CAD build for the part. Positions are in the model's coordinates, mm. A direction names the side the tool comes from. Coordinates: 2 decimals unless noted, no trailing zeros. Write each loop counter-clockwise with the first axis right and the second up, starting at its lowest first coordinate (ties: lowest second). Pieces come first, ordered by that corner, then holes. Notation, with made-up numbers: (-29.5, 58.25) - (25.5, 58.25) arc R34 ccw to (25.5, 91.25) - close; hole circle Ø10 at (11.5, 10). An arc over 180 degrees is marked (long way). Answer in a Markdown table with one row per item. Add a question column.
Q1. Band-saw the part on A-A (y = 30). List the corners of the cut face in (x, z), and give its area (3 significant figures).
Q2. Pin check, flat tip, straight feed: pin 1 (7.5 mm diameter, centred on x = 22.5, y = 19, fed in from +Z). Stop position of the tip, or through.
Q3. 3-axis set-ups, long thin cutter, end or side, ignore diameter. For faces 4 (the flat face through (0, 17, 2)), 5 (the flat face through (20, 11.5, 1)), 6 (the flat face through (20, 18, 0)), 7 (the cylindrical face through (7, 17, 2)), 8 (the flat face through (31.5, 15.4, 2.5)): which of +Z, -Z, +X, -X, +Y, -Y reach the whole face in a straight line?
Q4. Band-saw the part on C-C (z = 0.45). List the corners of the cut face in (x, y).
Q5. Drill centre lines: line 1 along X through (y, z) = (7, 3.1); line 2 along Y through (x, z) = (22.5, 2.7); line 3 along X through (y, z) = (16, 3.2). Where is each one in solid material? Low to high. Write a range as from..to.
Q6. Two-plate mould, pull along Y, no slides. Class faces 1 (the flat face through (41, 17, 2)), 2 (the cylindrical face through (39.859, 33.797, 2.028)), 3 (the flat face through (20, 19, 2)): +Y half, -Y half, draft (parallel to the pull), parting line (faces both ways), or undercut.
Q7. Band-saw the part on D-D (y = 25). List the corners of the cut face in (x, z), and give its area (3 significant figures).
Q8. Band-saw the part on B-B (x = 13.5). List the corners of the cut face in (y, z), and give its area (3 significant figures).
```python
from build123d import *

# Parameters (mm, degrees)
ESQUISSE1_W             = 41
ESQUISSE1_H             = 35
BOSS_EXTRU_1_DEPTH      = 4
ESQUISSE2_W             = 22
ESQUISSE2_H             = 18
ENL_V_MAT_EXTRU_1_DEPTH = 2
ESQUISSE3_W             = 4
ESQUISSE3_H             = 30
ESQUISSE3_W_2           = 22
ESQUISSE3_H_2           = 3
ENL_V_MAT_EXTRU_2_DEPTH = 6
CONG_4_R                = 4
CONG_6_RADIUS           = 2
CONG_6_LENGTH           = 30
CONG_7_RADIUS           = 2
CONG_7_LENGTH           = 30
CONG_8_RADIUS           = 2
CONG_8_LENGTH           = 30
CONG_9_RADIUS           = 2
CONG_9_LENGTH           = 30


with BuildPart() as part:
    # Esquisse1 → Boss.-Extru.1 (new body)
    with BuildSketch(Plane.XY):
        with Locations((20.5, 17.5)):
            Rectangle(ESQUISSE1_W, ESQUISSE1_H)
    extrude(amount=BOSS_EXTRU_1_DEPTH)

    # Esquisse2 → Enlèv. mat.-Extru.1 (cut)
    with BuildSketch(Plane.XY.offset(4)):
        with Locations((20.5, 17.5)):
            Rectangle(ESQUISSE2_W, ESQUISSE2_H)
    extrude(amount=-ENL_V_MAT_EXTRU_1_DEPTH, mode=Mode.SUBTRACT)

    # Esquisse3 → Enlèv. mat.-Extru.2 (cut)
    with BuildSketch(Plane.XY.offset(4)):
        with Locations((5, 17.5)):
            Rectangle(ESQUISSE3_W, ESQUISSE3_H)
        with Locations((36, 17.5)):
            Rectangle(ESQUISSE3_W, ESQUISSE3_H)
        with Locations((20.5, 10)):
            Rectangle(ESQUISSE3_W_2, ESQUISSE3_H_2)
    extrude(amount=-ENL_V_MAT_EXTRU_2_DEPTH, mode=Mode.SUBTRACT)

    # Congé4
    cong_4_edges = [part.edges().sort_by_distance(p)[0] for p in [
        (0, 35, 2),
        (41, 35, 2),
        (41, 0, 2),
        (0, 0, 2),
    ]]
    fillet(cong_4_edges, radius=CONG_4_R)

    # Congé6: full round fillet: the end face becomes a half cylinder, R = half its width
    cong_6_face = Plane((38, 17.5, 2), x_dir=(0, -1, 0), z_dir=(-1, 0, 0))  # on the end face: x along it, z out of the body
    cong_6_slab = cong_6_face.offset(-CONG_6_RADIUS / 2) * Box(CONG_6_LENGTH, 2 * CONG_6_RADIUS, CONG_6_RADIUS, mode=Mode.PRIVATE)  # the body's end, R deep
    cong_6_round = Plane((40, 17.5, 2), x_dir=(-1, 0, 0), z_dir=(0, -1, 0)) * Cylinder(CONG_6_RADIUS, CONG_6_LENGTH, mode=Mode.PRIVATE)  # its axis R under the face
    add(cong_6_slab - cong_6_round, mode=Mode.SUBTRACT)

    # Congé7: full round fillet: the end face becomes a half cylinder, R = half its width
    cong_7_face = Plane((3, 17.5, 2), x_dir=(0, 1, 0), z_dir=(1, 0, 0))  # on the end face: x along it, z out of the body
    cong_7_slab = cong_7_face.offset(-CONG_7_RADIUS / 2) * Box(CONG_7_LENGTH, 2 * CONG_7_RADIUS, CONG_7_RADIUS, mode=Mode.PRIVATE)  # the body's end, R deep
    cong_7_round = Plane((1, 17.5, 2), x_dir=(1, 0, 0), z_dir=(0, 1, 0)) * Cylinder(CONG_7_RADIUS, CONG_7_LENGTH, mode=Mode.PRIVATE)  # its axis R under the face
    add(cong_7_slab - cong_7_round, mode=Mode.SUBTRACT)

    # Congé8: full round fillet: the end face becomes a half cylinder, R = half its width
    cong_8_face = Plane((34, 17.5, 2), x_dir=(0, 1, 0), z_dir=(1, 0, 0))  # on the end face: x along it, z out of the body
    cong_8_slab = cong_8_face.offset(-CONG_8_RADIUS / 2) * Box(CONG_8_LENGTH, 2 * CONG_8_RADIUS, CONG_8_RADIUS, mode=Mode.PRIVATE)  # the body's end, R deep
    cong_8_round = Plane((32, 17.5, 2), x_dir=(1, 0, 0), z_dir=(0, 1, 0)) * Cylinder(CONG_8_RADIUS, CONG_8_LENGTH, mode=Mode.PRIVATE)  # its axis R under the face
    add(cong_8_slab - cong_8_round, mode=Mode.SUBTRACT)

    # Congé9: full round fillet: the end face becomes a half cylinder, R = half its width
    cong_9_face = Plane((7, 17.5, 2), x_dir=(0, -1, 0), z_dir=(-1, 0, 0))  # on the end face: x along it, z out of the body
    cong_9_slab = cong_9_face.offset(-CONG_9_RADIUS / 2) * Box(CONG_9_LENGTH, 2 * CONG_9_RADIUS, CONG_9_RADIUS, mode=Mode.PRIVATE)  # the body's end, R deep
    cong_9_round = Plane((9, 17.5, 2), x_dir=(-1, 0, 0), z_dir=(0, -1, 0)) * Cylinder(CONG_9_RADIUS, CONG_9_LENGTH, mode=Mode.PRIVATE)  # its axis R under the face
    add(cong_9_slab - cong_9_round, mode=Mode.SUBTRACT)


solid = part.part
```
Checked values:
| question | item | result |
|---|---|---|
| 1 | outline | (0, 0) - (1, 0) arc R2 ccw to (1, 4) - (0, 4) - close; (9, 0) - (32, 0) arc R2 ccw to (32, 4) - (9, 4) arc R2 ccw to start; (40, 0) - (41, 0) - (41, 4) - (40, 4) arc R2 ccw to start |
| 1 | area | 125 mm² |
| 2 | pin 1 | stops at z = 2 |
| 3 | face 4 | +Z, -Z, -X, +Y, -Y |
| 3 | face 5 | +Z, -Z |
| 3 | face 6 | -Z, +X, -X, +Y, -Y |
| 3 | face 7 | none |
| 3 | face 8 | +Z |
| 4 | outline | (0, 4) arc R4 ccw to (4, 0) - (37, 0) arc R4 ccw to (41, 4) - (41, 31) arc R4 ccw to (37, 35) - (4, 35) arc R4 ccw to (0, 31) - close; hole (2.26, 2.5) - (7.74, 2.5) - (7.74, 32.5) - (2.26, 32.5) - close; hole (9.5, 8.5) - (31.5, 8.5) - (31.5, 11.5) - (9.5, 11.5) - close; hole (33.26, 2.5) - (38.74, 2.5) - (38.74, 32.5) - (33.26, 32.5) - close |
| 5 | line 1 | x = 0..2.67, 7.33..33.67, 38.33..41 |
| 5 | line 2 | y = 0..8.5, 26.5..35 |
| 5 | line 3 | x = 0..2.6, 7.4..9.5, 31.5..33.6, 38.4..41 |
| 6 | face 1 | draft |
| 6 | face 2 | +Y half |
| 6 | face 3 | undercut |
| 7 | outline | (0, 0) - (1, 0) arc R2 ccw to (1, 4) - (0, 4) - close; (9, 0) - (32, 0) arc R2 ccw to (32, 4) - (31.5, 4) - (31.5, 2) - (9.5, 2) - (9.5, 4) - (9, 4) arc R2 ccw to start; (40, 0) - (41, 0) - (41, 4) - (40, 4) arc R2 ccw to start |
| 7 | area | 81.1 mm² |
| 8 | outline | (0, 0) - (8.5, 0) - (8.5, 4) - (0, 4) - close; (11.5, 0) - (35, 0) - (35, 4) - (26.5, 4) - (26.5, 2) - (11.5, 2) - close |
| 8 | area | 98.0 mm² |
